Autodesk Inventor part; units mm, degrees
ref_plane "YZ Plane" through (0, 0, 0) normal (1, 0, 0) x (0, 1, 0)
ref_plane "XZ Plane" through (0, 0, 0) normal (0, 1, 0) x (-1, 0, 0)
ref_plane "XY Plane" through (0, 0, 0) normal (0, 0, 1) x (1, 0, 0)
sketch "Sketch1" plane through (0, 0, 0) normal (0, 1, 0) x (-1, 0, 0)
  line L0 (-9.45, 13.9) -> (9.45, 13.9)
  line L1 (9.45, 13.9) -> (9.45, 12.4)
  line L2 (9.45, 12.4) -> (-9.45, 12.4)
  line L3 (-9.45, 12.4) -> (-9.45, 13.9)
  line L4 (9.45, 12.4) -> (6.45, 12.4)
  line L5 (6.45, 12.4) -> (6.45, -9)
  line L6 (6.45, -9) -> (9.45, -9)
  line L7 (9.45, -9) -> (9.45, 12.4)
  line L8 (-9.45, 12.4) -> (-7.95, 12.4)
  line L9 (-7.95, 12.4) -> (-7.95, -9)
  line L10 (-7.95, -9) -> (-9.45, -9)
  line L11 (-9.45, -9) -> (-9.45, 12.4)
  line L12 (-7.95, -7.6) -> (-9.45, -7.6)
  line L13 (-9.45, -7.6) -> (-9.45, -10.6)
  line L14 (-9.45, -10.6) -> (-7.95, -10.6)
  line L15 (-7.95, -10.6) -> (-7.95, -7.6)
  line L16 (1.45, -9) -> (9.45, -9)
  line L17 (9.45, -9) -> (9.45, -12)
  line L18 (9.45, -12) -> (1.45, -12)
  line L19 (1.45, -12) -> (1.45, -9)
  line L20 (-9.45, -10.6) -> (-7.95, -10.6)
  line L21 (-7.95, -10.6) -> (-7.95, -22.6)
  line L22 (-7.95, -22.6) -> (-9.45, -22.6)
  line L23 (-9.45, -22.6) -> (-9.45, -10.6)
  line L24 (9.45, -12) -> (6.45, -12)
  line L25 (6.45, -12) -> (6.45, -22.6)
  line L26 (6.45, -22.6) -> (9.45, -22.6)
  line L27 (9.45, -22.6) -> (9.45, -12)
  line L28 (-7.95, -22.6) -> (-19.45, -22.6)
  line L29 (-19.45, -22.6) -> (-19.45, -25.6)
  line L30 (-19.45, -25.6) -> (-7.95, -25.6)
  line L31 (-7.95, -25.6) -> (-7.95, -22.6)
  line L32 (6.45, -22.6) -> (19.45, -22.6)
  line L33 (19.45, -22.6) -> (19.45, -25.6)
  line L34 (19.45, -25.6) -> (6.45, -25.6)
  line L35 (6.45, -25.6) -> (6.45, -22.6)
  line L36 (-14.45, -26) -> (-14.45, -42) construction
  line L37 (14.45, -27) -> (14.45, -42) construction
  point P0 (0, 0)
  point P1 (0, 12.4)
  dimension "d0" = 1.5
  dimension "d1" = 3
  dimension "d2" = 1.5
  dimension "d3" = 3
  dimension "d4" = 3
  dimension "d5" = 0
  dimension "d6" = 5
  dimension "d7" = 14.4
  dimension "d8" = 21.4
  dimension "d9" = 20
  dimension "d12" = 0
  dimension "d13" = 0
  dimension "d20" = 12
  dimension "d21" = 10
  dimension "d22" = 1.5
  dimension "d23" = 3
  dimension "d24" = 10
  dimension "d25" = 3
  dimension "d26" = 3
  dimension "d33" = 5
  dimension "d34" = 5
  dimension "d35" = 28.9
extrude "Extrusion1" add sketch "Sketch1" along normal blind 10
sketch "Sketch6" plane through (19.45, 0, -25.6) normal (0, 0, -1) x (-1, 0, 0)
  line L0 (0, 10) -> (11.5, 10)
  line L1 (0, 0) -> (10, 0)
  line L2 (10, 0) -> (10, 10)
  line L3 (10, 10) -> (0, 10)
  line L4 (0, 10) -> (0, 0)
  circle A0 centre (5, 5) radius 2.25
  point P0 (19.45, 0)
  dimension "d27" = 4.5
sketch "Sketch7" plane through (-6.45, 0, -25.6) normal (0, 0, -1) x (-1, 0, 0)
  line L0 (0, 10) -> (13, 10)
  line L1 (13, 0) -> (3, 0)
  line L2 (3, 0) -> (3, 10)
  line L3 (3, 10) -> (13, 10)
  line L4 (13, 10) -> (13, 0)
  circle A0 centre (8, 5) radius 2.25
  point P0 (-6.45, 0)
  dimension "d28" = 4.5
extrude "Extrusion4" cut sketch "Sketch6" against normal blind 4 contours A0
extrude "Extrusion5" cut sketch "Sketch7" against normal blind 4 contours A0
sketch "Sketch8" plane through (0, 0, 0) normal (0, -1, 0) x (1, 0, 0)
  line L0 (2.9056, 13.9) -> (14.45, 13.9)
  line L1 (14.45, 13.9) -> (14.45, -22.6)
  line L2 (14.45, -22.6) -> (2.9056, -22.6)
  line L3 (2.9056, -22.6) -> (2.9056, 13.9)
  line L4 (9.45, -22.6) -> (19.45, -22.6)
  line L5 (-9.45, 13.9) -> (9.45, 13.9)
  point P0 (0, 0)
extrude "Extrusion6" cut sketch "Sketch8" against normal blind 5
equation "\"sp\" = 0.4"
properties part number "MotorMount"
Source: CAD feature listing. Evaluate the final solid. Frame: model axes, mm. A direction names the side the tool comes from. Round coordinates to 2 decimals unless told otherwise and drop trailing zeros. Loops run counter-clockwise (first coordinate to the right, second up) from the corner with the lowest first, then second, coordinate; pieces in that order, holes last.
Q1. Mould query, pull axis Y, two halves, no side actions, for faces 4 (the face through (-2.8, 10, -11.6)), 5 (the face through (12.304, 5.676, -24.121)), 6 (the face through (19.45, 5, -24)), 7 (the face through (14, 0, -24)). Classes: pulls with the +Y half, pulls with the -Y half, needs draft (parallel to the pull), parting line crosses it, or undercut.
Q2. First-contact query: P1, Ø5, axis at x = -14.45, y = 5, coming from the +Z side; P2, Ø4, axis at y = 8, z = -1, coming from the +X side; P3, Ø3, axis at y = 3.5, z = -20, coming from the -X side. Flat tips, straight axial feed; report the tip coordinate or a pass-through.
Q3. Section A-A, the plane x = -14.45. Return loops of the section in (y, z), plus the area to 3 significant figures.
Q4. Ray query, line 1 (X direction, y = 7.75, z = -21); line 2 (Y direction, x = -14.45, z = -24.75); line 3 (X direction, y = 7.5, z = -9.5). Return the intervals inside material, ascending.
Q5. Section B-B, the plane z = -19. Return loops of the section in (x, y), plus the area to 3 significant figures.
Q6. Access query for faces 1 (the face through (-6.45, 5, -19)), 2 (the face through (8.3, 5, -1.6)), 3 (the face through (-1, 5, 12.4)). Directions: +Z, -Z, +X, -X, +Y, -Y. A direction counts if a zero-diameter tool reaches every point of the face in a straight line with its end or side. Return the directions, or none.
Q7. Section C-C, the plane y = 9. Return loops of the section in (x, z), plus the area to 3 significant figures.
Q8. Section D-D, the plane y = 4.25. Return loops of the section in (x, z), plus the area to 3 significant figures.
Solutions:
1. face 4: pulls with the +Y half
1. face 5: undercut
1. face 6: needs draft
1. face 7: pulls with the -Y half
2. P1: stops at z = -22.6
2. P2: stops at x = 9.45
2. P3: stops at x = -9.45
3. outline: (0, -25.6) - (2.75, -25.6) - (2.75, -22.6) - (0, -22.6) - close; (7.25, -25.6) - (10, -25.6) - (10, -22.6) - (7.25, -22.6) - close
3. area: 16.5 mm2
4. line 1: x = -9.45 to -6.45, 7.95 to 9.45
4. line 2: y = 0 to 2.75, 7.25 to 10
4. line 3: x = -9.45 to -1.45, 7.95 to 9.45
5. outline: (-9.45, 0) - (-6.45, 0) - (-6.45, 10) - (-9.45, 10) - close; (7.95, 5) - (9.45, 5) - (9.45, 10) - (7.95, 10) - close
5. area: 37.5 mm2
6. face 1: -Z, +Y, -Y
6. face 2: +Z, +X, -Y
6. face 3: +Y, -Y
7. outline: (-19.45, -25.6) - (-6.45, -25.6) - (-6.45, -12) - (-1.45, -12) - (-1.45, -9) - (-6.45, -9) - (-6.45, 12.4) - (7.95, 12.4) - (7.95, -25.6) - (19.45, -25.6) - (19.45, -22.6) - (9.45, -22.6) - (9.45, 13.9) - (-9.45, 13.9) - (-9.45, -22.6) - (-19.45, -22.6) - close
7. area: 274 mm2
8. outline: (-19.45, -25.6) - (-16.57, -25.6) - (-16.57, -22.6) - (-19.45, -22.6) - close; (-12.33, -25.6) - (-6.45, -25.6) - (-6.45, -12) - (-1.45, -12) - (-1.45, -9) - (-6.45, -9) - (-6.45, 12.4) - (2.91, 12.4) - (2.91, 13.9) - (-9.45, 13.9) - (-9.45, -22.6) - (-12.33, -22.6) - close; (7.95, -25.6) - (12.33, -25.6) - (12.33, -22.6) - (7.95, -22.6) - close; (16.57, -25.6) - (19.45, -25.6) - (19.45, -22.6) - (16.57, -22.6) - close
8. area: 187 mm2
